```python
from build123d import *

# Parameters (mm, degrees)
F0_R      = 16
F1_DEPTH  = 15
F2_R      = 10
F3_DEPTH  = 4.5
F4_R      = 14
F4_R_2    = 8
F5_DEPTH  = 10
F6_R      = 6
F7_DEPTH  = 9
F8_R      = 5
F9_DEPTH  = 25
F10_R     = 8
F10_R_2   = 6
F11_DEPTH = 2
F12_R     = 2


with BuildPart() as f1:
    # F0 (on Top) → F1 (new body)
    with BuildSketch(Plane.XY):
        Circle(F0_R)
    extrude(amount=F1_DEPTH)

    # F2 (on face) → F3 (cut)
    with BuildSketch(Plane.XY.offset(15)):
        Circle(F2_R)
    extrude(amount=-F3_DEPTH, mode=Mode.SUBTRACT)

    # F4 (on face) → F5 (cut)
    with BuildSketch(Plane(origin=(0, 0, 0), x_dir=(1, 0, 0), z_dir=(0, 0, -1))):
        Circle(F4_R)
        Circle(F4_R_2, mode=Mode.SUBTRACT)
    extrude(amount=-F5_DEPTH, mode=Mode.SUBTRACT)

    # F6 (on face) → F7 (cut)
    with BuildSketch(Plane(origin=(0, 0, 0), x_dir=(1, 0, 0), z_dir=(0, 0, -1))):
        Circle(F6_R)
    extrude(amount=-F7_DEPTH, mode=Mode.SUBTRACT)

    # F8 (on face) → F9 (cut)
    with BuildSketch(Plane.XY.offset(10.5)):
        Circle(F8_R)
    extrude(amount=-F9_DEPTH, mode=Mode.SUBTRACT)

    # F10 (on face) → F11 (cut)
    with BuildSketch(Plane(origin=(0, 0, 0), x_dir=(1, 0, 0), z_dir=(0, 0, -1))):
        Circle(F10_R)
        Circle(F10_R_2, mode=Mode.SUBTRACT)
    extrude(amount=-F11_DEPTH, mode=Mode.SUBTRACT)

    # F12
    f12_edges = [f1.edges().sort_by_distance(p)[0] for p in [
        (-16, 0, 15),
        (-10, 0, 15),
    ]]
    fillet(f12_edges, radius=F12_R)


solid = f1.part
```
Model file for the job. Use its own axes, mm. A direction names the side the tool comes from. Give positions to 0.01 mm unless a question says otherwise; leave off trailing zeros. Order: outer loops, then holes, each group sorted by start corner. A loop starts at its lowest first (then second) coordinate and runs counter-clockwise, first axis right, second up.
1) Pin check, flat tips, straight feed: pin 1 (1.5 mm diameter, centred on x = 4, y = 8, fed in from +Z); pin 2 (6 mm diameter, centred on x = -3, z = 2, fed in from +Y); pin 3 (2 mm diameter, centred on x = 5.5, z = 4.5, fed in from -Y); pin 4 (9.5 mm diameter, centred on x = 3, y = -1.5, fed in from -Z). Stop position of each tip, or through.
2) Saw through at D-D, the plane z = 12.25. Write the cut outline in (x, y), then the cut area to 3 significant figures.
3) Saw through at A-A, the plane y = 0. Write the cut outline in (x, z), then the cut area to 3 significant figures.
4) 3-axis set-ups, long thin cutter, end or side, ignore diameter. For faces 1 (the cylindrical face through (-2.17, -9.76, 11.77)), 2 (the flat face through (-6.3, 10.4, 15)), 3 (the flat face through (-4, -4, 9)): which of +Z, -Z, +X, -X, +Y, -Y reach the whole face in a straight line?
5) Mould opens along Y. For faces 4 (the cylindrical face through (-3.47, -15.62, 6.41)), 5 (the flat face through (-0.07, -14.15, 0)), 6 (the cylindrical face through (-1.08, -4.88, 9.76)), 7 (the cylindrical face through (-1.73, 7.81, 5.94)) say: +Y half, -Y half, draft (parallel to the pull), parting line (faces both ways), or undercut.
6) Wall check: probe 1 along Y at (x, z) = (0, 7.5); probe 2 along Y at (x, z) = (0, 12.35); probe 3 along X at (y, z) = (7, 4). Give the ranges that are in metal, low to high.
7) Saw through at C-C, the plane z = 5.75. Write the cut outline in (x, y), then the cut area to 3 significant figures.
Computed:
1. pin 1: stops at z = 10.5
1. pin 2: stops at y = 16
1. pin 3: stops at y = -15.35
1. pin 4: stops at z = 2
2. outline: circle Ø32 at (0, 0); hole circle Ø20 at (0, 0)
2. area: 490 mm2
3. outline: (-16, 0) - (-14, 0) - (-14, 10) - (-8, 10) - (-8, 2) - (-6, 2) - (-6, 9) - (-5, 9) - (-5, 10.5) - (-10, 10.5) - (-10, 13) arc R2 ccw to (-12, 15) - (-14, 15) arc R2 ccw to (-16, 13) - close; (5, 9) - (6, 9) - (6, 2) - (8, 2) - (8, 10) - (14, 10) - (14, 0) - (16, 0) - (16, 13) arc R2 ccw to (14, 15) - (12, 15) arc R2 ccw to (10, 13) - (10, 10.5) - (5, 10.5) - close
3. area: 136 mm2
4. face 1: +Z
4. face 2: +Z, +X, -X, +Y, -Y
4. face 3: -Z
5. face 4: parting line
5. face 5: draft
5. face 6: undercut
5. face 7: undercut
6. probe 1: y = -16 to -14, -8 to -6, 6 to 8, 14 to 16
6. probe 2: y = -16 to -10, 10 to 16
6. probe 3: x = -14.39 to -12.12, -3.87 to 3.87, 12.12 to 14.39
7. outline: circle Ø32 at (0, 0); circle Ø16 at (0, 0); hole circle Ø28 at (0, 0); hole circle Ø12 at (0, 0)
7. area: 276 mm2
